from build123d import *

# Parameters (mm, degrees)
F1_DEPTH    = 1.5
F2_DEPTH    = 9
F0_W        = 4.5
F0_H        = 4.5
F0_R        = 1
F3_DEPTH    = 3.5
F0_W_2      = 16.5
F0_H_2      = 1.5
F4_DEPTH    = 5
F5_R        = 1.5
F6_DEPTH    = 3.5
F8_R        = 3
F9_W        = 0.6
F9_H        = 4
F9_W_2      = 1.5
F9_W_3      = 4
F9_H_2      = 0.6
F9_H_3      = 1.5
F10_DEPTH   = 1
F11_SIZE2   = 2
F11_SIZE    = 0.8
F11_2_SIZE2 = 2
F11_2_SIZE  = 0.8
F12_SIZE2   = 0.8
F12_SIZE    = 2


# Not quite as in the source:
# - a feature names something its author has since deleted; it is built from what else it names


with BuildPart() as f1:
    # F0 (on Top) → F1 (new body)
    with BuildSketch(Plane.XY):
        Polygon((8.2, 12.2), (-8.2, 12.2), (-8.2, 7.7), (-12.7, 7.7), (-12.7, -0.25), (-8.2, -0.25), (-8.2, -4.75), (-12.7, -4.75), (-12.7, -12.2), (-8.25, -12.2), (8.25, -12.2), (12.7, -12.2), (12.7, -4.75), (8.2, -4.75), (8.2, -0.25), (12.7, -0.25), (12.7, 7.7), (8.2, 7.7), align=None)
        Polygon((-6.5, 2), (-4.5, 2), (4.5, 2), (6.5, 2), (6.5, -9), (-6.5, -9), align=None, mode=Mode.SUBTRACT)
    extrude(amount=-F1_DEPTH)



with BuildPart() as f2:
    # F0 (on Top) → F2 (new body)
    with BuildSketch(Plane.XY):
        Polygon((-12.7, 7.7), (-12.7, 12.2), (-8.2, 12.2), (8.2, 12.2), (12.7, 12.2), (12.7, 7.7), (12.7, -0.25), (12.7, -4.75), (12.7, -12.2), (8.25, -12.2), (8.25, -13.7), (14.2, -13.7), (14.2, 13.7), (-14.2, 13.7), (-14.2, -13.7), (-8.25, -13.7), (-8.25, -12.2), (-12.7, -12.2), (-12.7, -4.75), (-12.7, -0.25), align=None)
    extrude(amount=-F2_DEPTH)


with BuildPart() as f3:
    # F0 (on Top) → F3 (new body)
    with BuildSketch(Plane.XY):
        with Locations((10.45, 9.95)):
            Rectangle(F0_W, F0_H)
        with Locations((10.5, 10)):
            Circle(F0_R, mode=Mode.SUBTRACT)
    extrude(amount=-F3_DEPTH)


with BuildPart() as f3b:
    # F0 (on Top) → F3, piece 2 (new body)
    with BuildSketch(Plane.XY):
        with Locations((10.45, -2.5)):
            Rectangle(F0_W, F0_H)
        with Locations((10.5, -2.5)):
            Circle(F0_R, mode=Mode.SUBTRACT)
    extrude(amount=-F3_DEPTH)


with BuildPart() as f3c:
    # F0 (on Top) → F3, piece 3 (new body)
    with BuildSketch(Plane.XY):
        Polygon((-4.5, -7), (-4.5, 2), (-6.5, 2), (-6.5, -9), (6.5, -9), (6.5, 2), (4.5, 2), (4.5, -7), align=None)
    extrude(amount=-F3_DEPTH)


with BuildPart() as f3d:
    # F0 (on Top) → F3, piece 4 (new body)
    with BuildSketch(Plane.XY):
        with Locations((-10.45, 9.95)):
            Rectangle(F0_W, F0_H)
        with Locations((-10.5, 10)):
            Circle(F0_R, mode=Mode.SUBTRACT)
    extrude(amount=-F3_DEPTH)


with BuildPart() as f3e:
    # F0 (on Top) → F3, piece 5 (new body)
    with BuildSketch(Plane.XY):
        with Locations((-10.45, -2.5)):
            Rectangle(F0_W, F0_H)
        with Locations((-10.5, -2.5)):
            Circle(F0_R, mode=Mode.SUBTRACT)
    extrude(amount=-F3_DEPTH)


with BuildPart() as f1_1:
    add(f1.part)

    add(f2.part)  # F4 merges F2
    # F0 (on Top) → F4 (join)
    with BuildSketch(Plane.XY):
        with Locations((0, -12.95)):
            Rectangle(F0_W_2, F0_H_2)
    extrude(amount=-F4_DEPTH)

    # F5 (on face) → F6 (join)
    with BuildSketch(Plane(origin=(-14.2, 0, 0), x_dir=(0, -1, 0), z_dir=(-1, 0, 0))):
        with Locations((11.2, -4.5)):
            Circle(F5_R)
        with Locations((-10.8, -4.5)):
            Circle(F5_R)
    extrude(amount=F6_DEPTH)



with BuildPart() as f1_2:
    add(f1_1.part)

    add(f3.part)  # F7 merges F3

    add(f3b.part)  # F7 merges F3b

    add(f3c.part)  # F7 merges F3c

    add(f3d.part)  # F7 merges F3d

    add(f3e.part)  # F7 merges F3e
    # F7: F1 across plane
    add(f1_1.part.mirror(Plane.YZ))

    # F8
    f8_edges = [f1_2.edges().sort_by_distance(p)[0] for p in [
        (8.2, 7.7, -2.5),
        (-8.2, 7.7, -2.5),
    ]]
    fillet(f8_edges, radius=F8_R)

    # F9 (on face) → F10 (join)
    with BuildSketch(Plane(origin=(0, 0, -9), x_dir=(1, 0, 0), z_dir=(0, 0, -1))):
        with Locations((-12.4, 8.7)):
            Rectangle(F9_W, F9_H)
        with Locations((-13.45, 8.7)):
            Rectangle(F9_W_2, F9_H)
        with Locations((12.4, 8.7)):
            Rectangle(F9_W, F9_H)
        with Locations((13.45, 8.7)):
            Rectangle(F9_W_2, F9_H)
        with Locations((0, -11.9)):
            Rectangle(F9_W_3, F9_H_2)
        with Locations((0, -12.95)):
            Rectangle(F9_W_3, F9_H_3)
    extrude(amount=F10_DEPTH)

    # F11
    f11_edges = [f1_2.edges().sort_by_distance(p)[0] for p in [
        (-12.1, -8.7, -10),
    ]]
    f11_side = f1_2.faces().sort_by_distance((-12.1, -8.7, -9.5))[0]
    chamfer(f11_edges, length=F11_SIZE, length2=F11_SIZE2, reference=f11_side)

    # F11#2
    f11_2_edges = [f1_2.edges().sort_by_distance(p)[0] for p in [
        (0, 11.6, -10),
    ]]
    f11_2_side = f1_2.faces().sort_by_distance((0, 11.6, -9.5))[0]
    chamfer(f11_2_edges, length=F11_2_SIZE, length2=F11_2_SIZE2, reference=f11_2_side)

    # F12
    f12_edges = [f1_2.edges().sort_by_distance(p)[0] for p in [
        (12.1, -8.7, -10),
    ]]
    f12_side = f1_2.faces().sort_by_distance((13.15, -8.7, -10))[0]
    chamfer(f12_edges, length=F12_SIZE, length2=F12_SIZE2, reference=f12_side)


solid = f1_2.part
Part model, mm, in its own coordinate system. A direction names the side the tool comes from. Coordinates: 2 decimals unless noted, no trailing zeros. Loops run counter-clockwise (first coordinate to the right, second up) from the corner with the lowest first, then second, coordinate; pieces in that order, holes last. Notation, with made-up numbers: (5.5, -11) - (49.5, -11) arc R24 ccw to (49.5, 19) - close; hole circle Ø3 at (19.25, 22.5). An arc over 180 degrees is marked (long way). Write each question's results on one line, items separated by ' | '. Start each with the question number.
Q1. Slice it at D-D on y = 10. Give the cut face in (x, z), and give its area (3 significant figures).
Q2. Which spindle directions (+Z, -Z, +X, -X, +Y, -Y) get a long thin tool onto all of the face, cutting with end or side? Do faces 4 (the flat face through (-13, 7, -9)), 5 (the flat face through (-8.25, -13, -7)), 6 (the flat face through (-13.4, -10.7, -9.4)), 7 (the flat face through (12.7, 0, -5)). Say none if no direction does.
Q3. Probe line 1 along Y through (x, z) = (-12.5, -2.5); line 2 along X through (y, z) = (-3.75, -1.75); line 3 along Y through (x, z) = (-10.5, -1.4). List the from-to ranges inside material, lowest first.
Q4. Two-plate mould, pull along X, no slides. Class faces 1 (the flat face through (0, -12.2, -4)), 2 (the flat face through (-12, -13, -9)), 3 (the flat face through (17.7, -11, -4)): +X half, -X half, draft (parallel to the pull), parting line (faces both ways), or undercut.
Q5. Slice it at A-A on z = -2.25. Give the number of separate pieces and of enclosed holes in the cut face, and give its area (3 significant figures).
Q6. Slice it at C-C on y = 1.25. Give the cut face in (x, z), and give its area (3 significant figures).
Q7. Drop flat-ended pins along their axis: pin 1 Ø1.6 at (y, z) = (-2, -3) entering from +X; pin 2 Ø3.5 at (x, y) = (9.5, 9.5) entering from -Z; pin 3 Ø13.5 at (x, y) = (-5.5, 6) entering from -Z. Give the stop position or say it passes through.
Q8. Slice it at B-B on x = 4. Give the cut face in (y, z), and give its area (3 significant figures).
Answer:
1) outline: (-17.7, -5.77) - (-14.2, -5.77) - (-14.2, -9) - (-12.7, -9) - (-12.7, -3.5) - (-11.5, -3.5) - (-11.5, 0) - (-14.2, 0) - (-14.2, -3.23) - (-17.7, -3.23) - close; (-9.5, -3.5) - (-8.28, -3.5) - (-8.28, -1.5) - (8.28, -1.5) - (8.28, -3.5) - (9.5, -3.5) - (9.5, 0) - (-9.5, 0) - close; (11.5, -3.5) - (12.7, -3.5) - (12.7, -9) - (14.2, -9) - (14.2, -5.77) - (17.7, -5.77) - (17.7, -3.23) - (14.2, -3.23) - (14.2, 0) - (11.5, 0) - close | area: 86.5 mm2
2) face 4: -Z, -X, +Y | face 5: -Z, -Y | face 6: -Z, +X, -X, -Y | face 7: none
3) line 1: y = -13.7 to -12.2, -4.75 to -0.25, 7.7 to 13.7 | line 2: x = -14.2 to -8.2, -6.5 to -4.5, 4.5 to 6.5, 8.2 to 14.2 | line 3: y = -13.7 to -3.5, -1.5 to 9, 11 to 13.7
4) face 1: undercut | face 2: draft | face 3: +X half
5) separate pieces: 2 | enclosed holes: 5 | area: 285 mm2
6) outline: (-14.2, -9) - (-12.7, -9) - (-12.7, -1.5) - (-6.5, -1.5) - (-6.5, -3.5) - (-4.5, -3.5) - (-4.5, 0) - (-14.2, 0) - close; (4.5, -3.5) - (6.5, -3.5) - (6.5, -1.5) - (12.7, -1.5) - (12.7, -9) - (14.2, -9) - (14.2, 0) - (4.5, 0) - close | area: 59.6 mm2
7) pin 1: stops at x = 14.2 | pin 2: stops at z = -3.5 | pin 3: stops at z = -9.27
8) outline: (-13.7, -5) - (-12.2, -5) - (-12.2, -1.5) - (-9, -1.5) - (-9, -3.5) - (-7, -3.5) - (-7, 0) - (-13.7, 0) - close; (2, -1.5) - (12.2, -1.5) - (12.2, -9) - (13.7, -9) - (13.7, 0) - (2, 0) - close | area: 48.1 mm2
